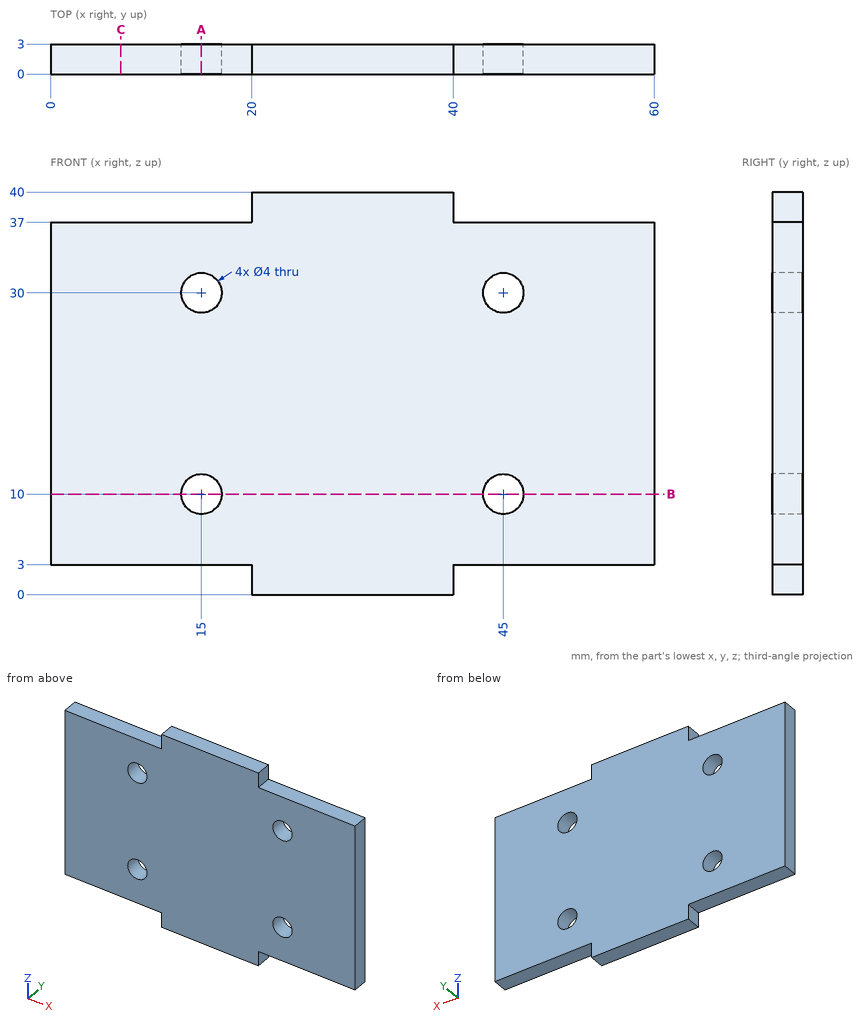
Job drawing, mm, ordinate dimensions from the low corner. One solid piece. Give positions to 0.01 mm unless a question says otherwise; leave off trailing zeros. Write each loop counter-clockwise with the first axis right and the second up, starting at its lowest first coordinate (ties: lowest second). Pieces come first, ordered by that corner, then holes. Notation, with made-up numbers: M 44.5,30.5 L 102.5,30.5 A21 ccw 102.5,62.5 Z; hole C 88,24.25 d5. An arc over 180 degrees is marked long. One line per item, written item: value. Start each with the question number.
Q1. Saw through at A-A, the plane x = 15. Write the cut outline in (y, z), plus the area to 3 significant figures.
Q2. Saw through at C-C, the plane x = 7. Write the cut outline in (y, z), plus the area to 3 significant figures.
Q3. Saw through at B-B, the plane z = 10. Write the cut outline in (x, y), plus the area to 3 significant figures.
Q4. Drop flat-ended pins along their axis: pin 1 Ø1.5 at (x, y) = (54.5, 1.5) entering from -Z; pin 2 Ø0.9 at (y, z) = (1, 38.5) entering from +X; pin 3 Ø1.5 at (y, z) = (2, 39) entering from -X. Give the stop position or say it passes through.
Q5. Probe probe 1 along X at (y, z) = (1.9, 30); probe 2 along X at (y, z) = (1.9, 9.5); probe 3 along Z at (x, y) = (5, 1.2). List the from-to ranges inside material, lowest first. Write a range as [from, to].
Output values:
1. outline: M 0,3 L 3,3 L 3,8 L 0,8 Z; M 0,12 L 3,12 L 3,28 L 0,28 Z; M 0,32 L 3,32 L 3,37 L 0,37 Z
1. area: 78.0 mm²
2. outline: M 0,3 L 3,3 L 3,37 L 0,37 Z
2. area: 102 mm²
3. outline: M 0,0 L 13,0 L 13,3 L 0,3 Z; M 17,0 L 43,0 L 43,3 L 17,3 Z; M 47,0 L 60,0 L 60,3 L 47,3 Z
3. area: 156 mm²
4. pin 1: stops at z = 3
4. pin 2: stops at x = 40
4. pin 3: stops at x = 20
5. probe 1: x = [0, 13], [17, 43], [47, 60]
5. probe 2: x = [0, 13.06], [16.94, 43.06], [46.94, 60]
5. probe 3: z = [3, 37]
